Check sheet for the drawn part. Datum: minimum x, y, z corner. Units: mm. A direction names the side the tool comes from. Round coordinates to 2 decimals unless told otherwise and drop trailing zeros. Order: outer loops, then holes, each group sorted by start corner. A loop starts at its lowest first (then second) coordinate and runs counter-clockwise, first axis right, second up. Notation, with made-up numbers: (9.5, 19) -> (66.5, 19) arc R25 cw to (66.5, 39) -> close; hole circle Ø10 at (-36.75, 75.5). An arc over 180 degrees is marked (long way). Use CSV: the item, a comma, the result in double quotes.
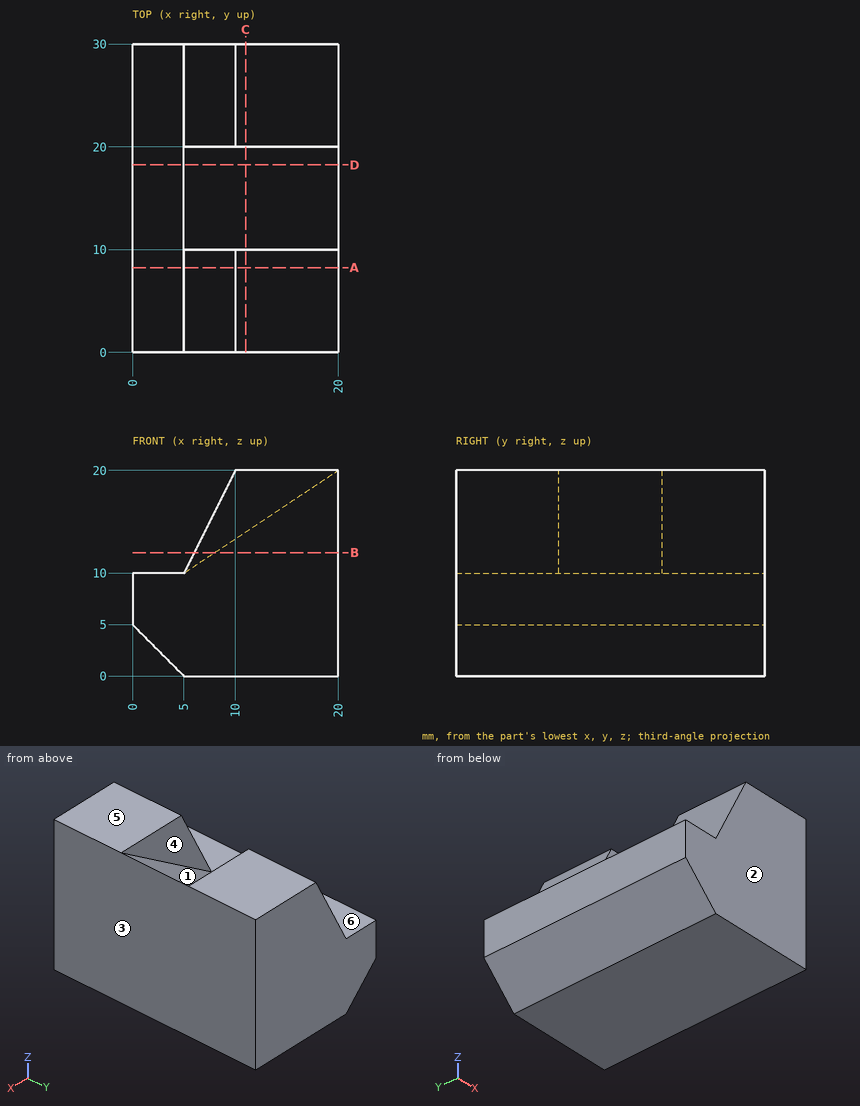
Q1. Access from +Z, -Z, +X, -X, +Y, -Y to the whole of each face (thin tool, end or side, straight path). Record for the marked faces 4, 5 and 6.
Result sheet:
face 4,"+Z, -X"
face 5,"+Z, +X, -X, +Y, -Y"
face 6,"+Z, -X, +Y, -Y"
Q2. Sectioned sample at A-A, the plane y = 8.25. Enter the section's corners in (x, z), then the cut area to 4 significant figures.
Result sheet:
outline,"(0, 5) -> (5, 0) -> (20, 0) -> (20, 20) -> (10, 20) -> (5, 10) -> (0, 10) -> close"
area,"312.5 mm^2"
Q3. Sectioned sample at C-C, the plane x = 11. Enter the section's corners in (y, z).
Result sheet:
outline,"(0, 0) -> (30, 0) -> (30, 20) -> (20, 20) -> (20, 14) -> (10, 14) -> (10, 20) -> (0, 20) -> close"
Q4. Scan lines: L1, parallel to X at y = 24.25, z = 17.25 (3 decimals); L2, parallel to X at y = 8, z = 3.5; L3, parallel to Z at x = 19.25, y = 15.5. Record each from-to range of solid material in increasing order.
Result sheet:
L1,"x = 8.625 to 20"
L2,"x = 1.5 to 20"
L3,"z = 0 to 19.5"
Q5. Sectioned sample at B-B, the plane z = 12. Enter the section's corners in (x, y), then the cut area to 3 significant figures.
Result sheet:
outline,"(6, 0) -> (20, 0) -> (20, 30) -> (6, 30) -> (6, 20) -> (8, 20) -> (8, 10) -> (6, 10) -> close"
area,"400 mm^2"
Q6. Go/stop test with flat-tipped pins: pin 1 (12 mm diameter, centred on y = 4, z = 17, fed in from -X); pin 2 (2.5 mm diameter, centred on x = 3, y = 20, fed in from +Z). Record where each tip stops, or that it passes through.
Result sheet:
pin 1,"stops at x = 5.5"
pin 2,"stops at z = 10"
Q7. Mould release check, pull along Y, two halves, no side actions. Record for the marked faces 1, 2 and 3: pulls with the +Y half, pulls with the -Y half, needs draft (parallel to the pull), parting line crosses it, or undercut.
Result sheet:
face 1,"undercut"
face 2,"pulls with the -Y half"
face 3,"needs draft"
Q8. Sectioned sample at D-D, the plane y = 18.25. Enter the section's corners in (x, z).
Result sheet:
outline,"(0, 5) -> (5, 0) -> (20, 0) -> (20, 20) -> (5, 10) -> (0, 10) -> close"
